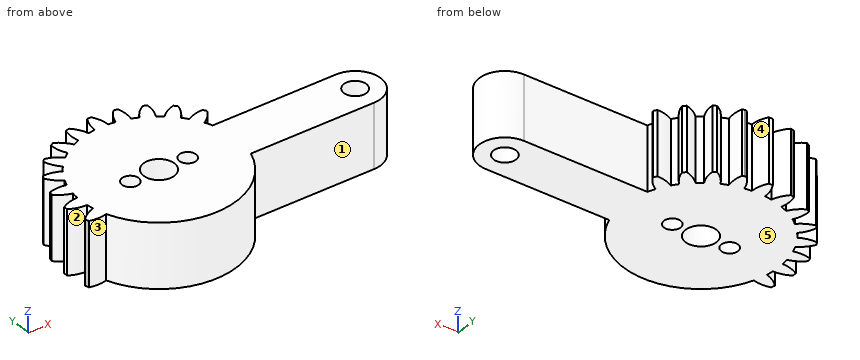
Autodesk Fusion 360 part; units mm, degrees
sketch "Sketch1" plane through (0, 0, 0) normal (0, 0, 1) x (1, 0, 0)
  circle A0 centre (0, 0) radius 12.09
  line L0 (0, 0) -> (30.75, 0)
  circle A1 centre (30.75, 0) radius 1.75
  circle A2 centre (0, 0) radius 1.75
  line L1 (0, -14.63) -> (0, 14.63) construction
  line L2 (0, 14.63) -> (-0.31, 14.63)
  line L3 (0, 14.63) -> (-0.31, 14.63)
  arc A3 (-0.31, 14.63) -> (-1.04, 12.0452) centre (3.9012, 12.0452) ccw
  arc A4 (1.04, 12.0452) -> (0.31, 14.63) centre (-3.9012, 12.0452) ccw
  line L4 (0.31, 14.63) -> (0, 14.63)
  arc A5 (-4.086, 14.0513) -> (-4.1221, 11.3656) centre (0.6508, 12.6445) ccw
  line L5 (-3.7865, 14.1315) -> (-4.086, 14.0513)
  line L6 (-3.4871, 14.2117) -> (-3.7865, 14.1315)
  arc A6 (-2.113, 11.9039) -> (-3.4871, 14.2117) centre (-6.8858, 10.625) ccw
  arc A7 (-7.5835, 12.515) -> (-6.9233, 9.9114) centre (-2.644, 12.382) ccw
  line L7 (-7.315, 12.67) -> (-7.5835, 12.515)
  line L8 (-7.0465, 12.825) -> (-7.315, 12.67)
  arc A8 (-5.1219, 10.9514) -> (-7.0465, 12.825) centre (-9.4011, 8.4808) ccw
  arc A9 (-10.5642, 10.1258) -> (-9.2526, 7.7818) centre (-5.7587, 11.2758) ccw
  line L9 (-10.345, 10.345) -> (-10.5642, 10.1258)
  line L10 (-10.1258, 10.5642) -> (-10.345, 10.345)
  arc A10 (-7.7818, 9.2526) -> (-10.1258, 10.5642) centre (-11.2758, 5.7587) ccw
  arc A11 (-12.825, 7.0465) -> (-10.9514, 5.1219) centre (-8.4808, 9.4011) ccw
  line L11 (-12.67, 7.315) -> (-12.825, 7.0465)
  line L12 (-12.515, 7.5835) -> (-12.67, 7.315)
  arc A12 (-9.9114, 6.9233) -> (-12.515, 7.5835) centre (-12.382, 2.644) ccw
  arc A13 (-14.2117, 3.4871) -> (-11.9039, 2.113) centre (-10.625, 6.8858) ccw
  line L13 (-14.1315, 3.7865) -> (-14.2117, 3.4871)
  line L14 (-14.0513, 4.086) -> (-14.1315, 3.7865)
  arc A14 (-11.3656, 4.1221) -> (-14.0513, 4.086) centre (-12.6445, -0.6508) ccw
  arc A15 (-14.63, -0.31) -> (-12.0452, -1.04) centre (-12.0452, 3.9012) ccw
  line L15 (-14.63, 0) -> (-14.63, -0.31)
  line L16 (-14.63, 0.31) -> (-14.63, 0)
  arc A16 (-12.0452, 1.04) -> (-14.63, 0.31) centre (-12.0452, -3.9012) ccw
  arc A17 (-14.0513, -4.086) -> (-11.3656, -4.1221) centre (-12.6445, 0.6508) ccw
  line L17 (-14.1315, -3.7865) -> (-14.0513, -4.086)
  line L18 (-14.2117, -3.4871) -> (-14.1315, -3.7865)
  arc A18 (-11.9039, -2.113) -> (-14.2117, -3.4871) centre (-10.625, -6.8858) ccw
  arc A19 (12.515, 7.5835) -> (9.9114, 6.9233) centre (12.382, 2.644) ccw
  line L19 (12.67, 7.315) -> (12.515, 7.5835)
  line L20 (12.825, 7.0465) -> (12.67, 7.315)
  arc A20 (10.9514, 5.1219) -> (12.825, 7.0465) centre (8.4808, 9.4011) ccw
  arc A21 (10.1258, 10.5642) -> (7.7818, 9.2526) centre (11.2758, 5.7587) ccw
  line L21 (10.345, 10.345) -> (10.1258, 10.5642)
  line L22 (10.5642, 10.1258) -> (10.345, 10.345)
  arc A22 (9.2526, 7.7818) -> (10.5642, 10.1258) centre (5.7587, 11.2758) ccw
  arc A23 (7.0465, 12.825) -> (5.1219, 10.9514) centre (9.4011, 8.4808) ccw
  line L23 (7.315, 12.67) -> (7.0465, 12.825)
  line L24 (7.5835, 12.515) -> (7.315, 12.67)
  arc A24 (6.9233, 9.9114) -> (7.5835, 12.515) centre (2.644, 12.382) ccw
  arc A25 (3.4871, 14.2117) -> (2.113, 11.9039) centre (6.8858, 10.625) ccw
  line L25 (3.7865, 14.1315) -> (3.4871, 14.2117)
  line L26 (4.086, 14.0513) -> (3.7865, 14.1315)
  arc A26 (4.1221, 11.3656) -> (4.086, 14.0513) centre (-0.6508, 12.6445) ccw
  circle A27 centre (30.75, 0) radius 4
  line L27 (30.75, 4) -> (11.4091, 4)
  line L28 (30.75, -4) -> (11.4091, -4)
  dimension "d1" = 24.18
  dimension "d2" = 30.75
  dimension "d3" = 3.5
  dimension "d4" = 3.5
  dimension "d5" = 29.26
  dimension "d6" = 0.31
  dimension "d9" = 360
  dimension "d10" = 8
extrude "Extrude1" add sketch "Sketch1" along normal blind 10
sketch "Sketch2" plane through (0, 0, 10) normal (0, 0, 1) x (-1, 0, 0)
  circle A0 centre (-30.75, 0) radius 1.75
  circle A1 centre (0, 0) radius 1.75
  line L0 (-30.75, -4) -> (-11.4091, -4)
  arc A2 (-11.4091, -4) -> (-10.9514, -5.1219) centre (0, 0) ccw
  arc A3 (-10.9514, -5.1219) -> (-12.825, -7.0465) centre (-8.4808, -9.4011) ccw
  line L1 (-12.825, -7.0465) -> (-12.515, -7.5835)
  arc A4 (-12.515, -7.5835) -> (-9.9114, -6.9233) centre (-12.382, -2.644) ccw
  arc A5 (-9.9114, -6.9233) -> (-9.2526, -7.7818) centre (0, 0) ccw
  arc A6 (-9.2526, -7.7818) -> (-10.5642, -10.1258) centre (-5.7587, -11.2758) ccw
  line L2 (-10.5642, -10.1258) -> (-10.1258, -10.5642)
  arc A7 (-10.1258, -10.5642) -> (-7.7818, -9.2526) centre (-11.2758, -5.7587) ccw
  arc A8 (-7.7818, -9.2526) -> (-6.9233, -9.9114) centre (0, 0) ccw
  arc A9 (-6.9233, -9.9114) -> (-7.5835, -12.515) centre (-2.644, -12.382) ccw
  line L3 (-7.5835, -12.515) -> (-7.0465, -12.825)
  arc A10 (-7.0465, -12.825) -> (-5.1219, -10.9514) centre (-9.4011, -8.4808) ccw
  arc A11 (-5.1219, -10.9514) -> (-4.1221, -11.3656) centre (0, 0) ccw
  arc A12 (-4.1221, -11.3656) -> (-4.086, -14.0513) centre (0.6508, -12.6445) ccw
  line L4 (-4.086, -14.0513) -> (-3.4871, -14.2117)
  arc A13 (-3.4871, -14.2117) -> (-2.113, -11.9039) centre (-6.8858, -10.625) ccw
  arc A14 (-2.113, -11.9039) -> (-1.04, -12.0452) centre (0, 0) ccw
  arc A15 (-1.04, -12.0452) -> (-0.31, -14.63) centre (3.9012, -12.0452) ccw
  line L5 (-0.31, -14.63) -> (0.31, -14.63)
  arc A16 (0.31, -14.63) -> (1.04, -12.0452) centre (-3.9012, -12.0452) ccw
  arc A17 (1.04, -12.0452) -> (2.113, -11.9039) centre (0, 0) ccw
  arc A18 (2.113, -11.9039) -> (3.4871, -14.2117) centre (6.8858, -10.625) ccw
  line L6 (3.4871, -14.2117) -> (4.086, -14.0513)
  arc A19 (4.086, -14.0513) -> (4.1221, -11.3656) centre (-0.6508, -12.6445) ccw
  arc A20 (4.1221, -11.3656) -> (5.1219, -10.9514) centre (0, 0) ccw
  arc A21 (5.1219, -10.9514) -> (7.0465, -12.825) centre (9.4011, -8.4808) ccw
  line L7 (7.0465, -12.825) -> (7.5835, -12.515)
  arc A22 (7.5835, -12.515) -> (6.9233, -9.9114) centre (2.644, -12.382) ccw
  arc A23 (6.9233, -9.9114) -> (7.7818, -9.2526) centre (0, 0) ccw
  arc A24 (7.7818, -9.2526) -> (10.1258, -10.5642) centre (11.2758, -5.7587) ccw
  line L8 (10.1258, -10.5642) -> (10.5642, -10.1258)
  arc A25 (10.5642, -10.1258) -> (9.2526, -7.7818) centre (5.7587, -11.2758) ccw
  arc A26 (9.2526, -7.7818) -> (9.9114, -6.9233) centre (0, 0) ccw
  arc A27 (9.9114, -6.9233) -> (12.515, -7.5835) centre (12.382, -2.644) ccw
  line L9 (12.515, -7.5835) -> (12.825, -7.0465)
  arc A28 (12.825, -7.0465) -> (10.9514, -5.1219) centre (8.4808, -9.4011) ccw
  arc A29 (10.9514, -5.1219) -> (11.3656, -4.1221) centre (0, 0) ccw
  arc A30 (11.3656, -4.1221) -> (14.0513, -4.086) centre (12.6445, 0.6508) ccw
  line L10 (14.0513, -4.086) -> (14.2117, -3.4871)
  arc A31 (14.2117, -3.4871) -> (11.9039, -2.113) centre (10.625, -6.8858) ccw
  arc A32 (11.9039, -2.113) -> (12.0452, -1.04) centre (0, 0) ccw
  arc A33 (12.0452, -1.04) -> (14.63, -0.31) centre (12.0452, 3.9012) ccw
  line L11 (14.63, -0.31) -> (14.63, 0.31)
  arc A34 (14.63, 0.31) -> (12.0452, 1.04) centre (12.0452, -3.9012) ccw
  arc A35 (12.0452, 1.04) -> (11.9039, 2.113) centre (0, 0) ccw
  arc A36 (11.9039, 2.113) -> (14.2117, 3.4871) centre (10.625, 6.8858) ccw
  line L12 (14.2117, 3.4871) -> (14.0513, 4.086)
  arc A37 (14.0513, 4.086) -> (11.3656, 4.1221) centre (12.6445, -0.6508) ccw
  arc A38 (11.3656, 4.1221) -> (-11.4091, 4) centre (0, 0) ccw
  line L13 (-11.4091, 4) -> (-30.75, 4)
  arc A39 (-30.75, 4) -> (-30.75, -4) centre (-30.75, 0) ccw
  line L14 (4.5, 0) -> (-4.5, 0) construction
  circle A40 centre (4.5, 0) radius 1.3
  circle A41 centre (-4.5, 0) radius 1.3
  dimension "d13" = 9
  dimension "d14" = 2.6
  dimension "d15" = 2.6
sketch "Sketch3" plane through (0, 0, 10) normal (0, 0, 1) x (-1, 0, 0)
extrude "Extrude2" cut sketch "Sketch2" against normal blind 10 contours A40
extrude "Extrude3" cut sketch "Sketch2" against normal blind 10 contours A41
sketch "Sketch4" plane through (0, 0, 10) normal (0, 0, 1) x (-1, 0, 0)
  circle A0 centre (0, 0) radius 2.4
  dimension "d20" = 4.8
extrude "Extrude4" cut sketch "Sketch4" against normal blind 10
Geometry check sheet. Reference: the model listing, model coordinates, mm. Face numbers are marked on the shaded views. A direction names the side the tool comes from. Coordinates: 2 decimals unless noted, no trailing zeros. Order: outer loops, then holes, each group sorted by start corner. A loop starts at its lowest first (then second) coordinate and runs counter-clockwise, first axis right, second up. Notation, with made-up numbers: M 12,-31 L 39,-31 A19 ccw 39,-6 Z; hole C 44.5,-7 d5. An arc over 180 degrees is marked long. Answer as a JSON object with one key per item and string values.
Q1. Tool access check on the marked faces 4 and 5. Record the directions out of +Z, -Z, +X, -X, +Y, -Y that give a thin tool (end or side, any length) a straight path to the whole face; none if there is none.
Results are:
{"face 4": "+Z, -Z, +Y", "face 5": "-Z, +X, -X, +Y, -Y"}
Q2. Release check for a two-part mould opening along X. For the marked faces 1, 2 and 3 record: released by +X, released by -X, zero draft, split by the parting line, or undercut.
Results are:
{"face 1": "zero draft", "face 2": "released by -X", "face 3": "undercut"}
Q3. Scan lines: line 1 (X direction, y = 0, z = 3.5); line 2 (Y direction, x = 30.75, z = 4.75); line 3 (X direction, y = 0.5, z = 6). Record each from-to range of solid material in increasing order.
Results are:
{"line 1": "x = -14.63 to -5.8, -3.2 to -2.4, 2.4 to 3.2, 5.8 to 29, 32.5 to 34.75", "line 2": "y = -4 to -1.75, 1.75 to 4", "line 3": "x = -14.29 to -5.7, -3.3 to -2.35, 2.35 to 3.3, 5.7 to 29.07, 32.43 to 34.72"}
Q4. Cross-section at A-A on x = 18. Record the cut outline in (y, z), and give its area (3 significant figures).
Results are:
{"outline": "M -4,0 L 4,0 L 4,10 L -4,10 Z", "area": "80.0 mm²"}
Q5. Depth check by flat-ended pin: pin 1 Ø3 at (x, y) = (-4.5, 0) entering from +Z; pin 2 Ø3 at (x, z) = (9, 5.5) entering from +Y; pin 3 Ø1 at (x, z) = (25, 7.5) entering from -Y; pin 4 Ø4 at (y, z) = (-3.5, 1) entering from -X. Enter the tip coordinate at first touch or a pass-through.
Results are:
{"pin 1": "stops at z = 10", "pin 2": "stops at y = 12.56", "pin 3": "stops at y = -4", "pin 4": "stops at x = -14.21"}
Q6. Cross-section at B-B on z = 8.25. Give the number of separate pieces and of enclosed holes in the cut face, and give its area (3 significant figures).
Results are:
{"separate pieces": "1", "enclosed holes": "4", "area": "646 mm²"}
Q7. Cross-section at C-C on y = -7.5. Record the cut outline in (x, z).
Results are:
{"outline": "M -9.48,0 L 9.48,0 L 9.48,10 L -9.48,10 Z"}
